Part model, mm, in its own coordinate system. Give positions to 0.01 mm unless a question says otherwise; leave off trailing zeros. Order: outer loops, then holes, each group sorted by start corner. A loop starts at its lowest first (then second) coordinate and runs counter-clockwise, first axis right, second up. Notation, with made-up numbers: M -33,7 L -4,7 A34 cw -4,40 Z; hole C 41.5,37.25 d8. An arc over 180 degrees is marked long. One line per question, with ' | ' between items.
```python
from build123d import *

# Parameters (mm, degrees)
SCHIZZO1_W               = 205
SCHIZZO1_H               = 1
SCHIZZO2_R               = 1.5
TAGLIO_ESTRUSIONE1_DEPTH = 10
SCHIZZO3_R               = 1
TAGLIO_ESTRUSIONE2_DEPTH = 10
RACCORDO4_R              = 0.5


with BuildPart() as part:
    # Schizzo1 → Rivoluzione1 (revolve)
    with BuildSketch(Plane(origin=(0, 0, 0), x_dir=(0, 0, -1), z_dir=(1, 0, 0)), mode=Mode.PRIVATE) as rivoluzione1_sk:
        with Locations((-22.156399009, 4.5)):
            Rectangle(SCHIZZO1_W, SCHIZZO1_H)
    revolve(rivoluzione1_sk.sketch.rotate(Axis((0, 0, 65.406887886), (0, 0, -1)), 90), axis=Axis((0, 0, 65.406887886), (0, 0, -1)))

    # Schizzo2 → Taglio-Estrusione1 (cut)
    with BuildSketch(Plane(origin=(0, 0, 0), x_dir=(1, 0, 0), z_dir=(0, 1, 0))):
        with Locations(Location((0, 64.343600991, 0), (0, 0, 270))):
            Circle(SCHIZZO2_R)
    extrude(amount=-TAGLIO_ESTRUSIONE1_DEPTH, mode=Mode.SUBTRACT)

    # Schizzo3 → Taglio-Estrusione2 (cut)
    with BuildSketch(Plane(origin=(0, 0, 0), x_dir=(0, 0, -1), z_dir=(1, 0, 0))):
        with Locations((65.343600991, 0)):
            Circle(SCHIZZO3_R)
    extrude(amount=-TAGLIO_ESTRUSIONE2_DEPTH, mode=Mode.SUBTRACT)

    # Raccordo4
    raccordo4_edges = [part.edges().sort_by_distance(p)[0] for p in [
        (-5, 0, -80.343600991),
        (-4, 0, -80.343600991),
    ]]
    fillet(raccordo4_edges, radius=RACCORDO4_R - 0.0001)  # a hair under: the kernel refuses the full size


solid = part.part
```
1. Mould opens along X. For faces 1 (the cylindrical face through (-5, 0, 21)), 2 (the cylindrical face through (-0.867, 3.905, 20.975)) say: released by +X, released by -X, zero draft, split by the parting line, or undercut.
Worked out:
face 1: split by the parting line | face 2: undercut
2. Drop flat-ended pins along their axis: pin 1 (1 mm diameter, centred on y = 1, z = 75, fed in from +X); pin 2 (1 mm diameter, centred on y = 4, z = 45.5, fed in from +X); pin 3 (3 mm diameter, centred on x = 0.5, y = 1, fed in from -Z). Give the stop position or say it passes through.
Worked out:
pin 1: stops at x = 4.97 | pin 2: stops at x = 3.57 | pin 3: passes through
3. Probe L1, parallel to Y at x = 0, z = -14; L2, parallel to X at y = 0.75, z = 73; L3, parallel to X at y = -0.5, z = -9. List the from-to ranges inside material, lowest first. Write a range as from..to.
Worked out:
L1: y = -5..-4, 4..5 | L2: x = -4.94..-3.93, 3.93..4.94 | L3: x = -4.97..-3.97, 3.97..4.97
4. Slice it at A-A on z = -61. Give the cut face in (x, y), then the cut area to 3 significant figures.
Worked out:
outline: C 0,0 d10; hole C 0,0 d8 | area: 28.3 mm2
